Autodesk Inventor part; units mm, degrees
ref_plane "YZ Plane" through (0, 0, 0) normal (1, 0, 0) x (0, 1, 0)
ref_plane "XZ Plane" through (0, 0, 0) normal (0, 1, 0) x (-1, 0, 0)
ref_plane "XY Plane" through (0, 0, 0) normal (0, 0, 1) x (1, 0, 0)
sketch "Sketch1" plane through (0, 0, 0) normal (1, 0, 0) x (0, 1, 0)
  line L0 (0, 0) -> (-4.0897, 0)
  line L1 (0, -1.6442) -> (0, -13.25)
  line L2 (0, -13.25) -> (3.5, -13.25)
  line L3 (3.5, -13.25) -> (3.5, -10.75)
  line L4 (3.5, -10.75) -> (0.5, -10.75)
  line L5 (4, 0) -> (4, -10)
  line L6 (4, -10) -> (0.5, -10)
  line L7 (0.5, -10) -> (0.5, -10.75)
  line L8 (3.5, -1.5) -> (3.5, -9.5)
  line L9 (3.5, -9.5) -> (0, -9.5)
  line L10 (3, -11.25) -> (0, -11.25)
  line L11 (3, -11.25) -> (3, -12.25)
  line L12 (3, -12.25) -> (0, -12.25)
  line L13 (3.5, -1.5) -> (4, -1.5)
  point P0 (1.5, -12.25)
  point P1 (3.75, -1.5)
  dimension "d1" = 26.5
  dimension "d2" = 2.5
  dimension "d3" = 3.5
  dimension "d4" = 0
  dimension "d5" = 4
  dimension "d6" = 20
  dimension "d7" = 0.5
  dimension "d8" = 0.5
  dimension "d9" = 0.5
  dimension "d10" = 0.5
  dimension "d11" = 0.5
  dimension "d12" = 1
  dimension "d13" = 3
revolve "Revolution1" add sketch "Sketch1" angle 360 about axis through (0, 0, 0) along (0, -1, 0) contours L9 L8 L13 L5 L6 L7 L4 L3 L2 L1 L12 L11 L10
sketch "Sketch2" plane through (0, 4, 0) normal (0, 1, 0) x (1, 0, 0)
  line L0 (-7.75, 0) -> (7.75, 0)
  point P0 (0, 0)
  point P1 (0, 0)
  dimension "d15" = 15.5
hole "Hole1" at (-7.75, 4, 0) at (7.75, 4, 0) direction (0, -1, 0) diameter 1.5 end through all
fillet "Fillet1" radius 0.6 2 edges at (0, 0, 11.25) (0, 0, 9.5)
equation "\"d8\" = d7"
equation "\"d9\" = d7"
equation "\"d10\" = d7"
equation "\"d11\" = d7"
properties part number "Diaphram" material "Rubber, Silicone"
Can you work these out from the model? Positions are in its coordinate system, mm. A direction names the side the tool comes from. Coordinates: 2 decimals unless noted, no trailing zeros. Loops run counter-clockwise (first coordinate to the right, second up) from the corner with the lowest first, then second, coordinate; pieces in that order, holes last. Notation, with made-up numbers: M -40,47.25 L -33,47.25 A12 ccw -33,63.25 Z; hole C -23.5,41.5 d3. An arc over 180 degrees is marked long. Put each result on its own line as item: value. Start each with the question number.
(1) Will these pins go through, and if not, where does the flat tip stop? pin 1 Ø1.5 at (x, y) = (5, 0.5) entering from +Z; pin 2 Ø2.5 at (x, z) = (-7.75, 0) entering from -Y; pin 3 Ø2.5 at (x, z) = (0, 0) entering from +Y; pin 4 Ø1.5 at (x, y) = (1, 2) entering from -Z.
(2) We'd pull the mould along Z, two halves only. Please class faces 4 (the face through (-9.76, 2.23, 2.17)), 5 (the face through (0, 4, -2)), 6 (the face through (-11.172, 1.774, -7.123)): +Z half, -Z half, draft (parallel to the pull), parting line (faces both ways), or undercut.
(3) Which directions (+Z, -Z, +X, -X, +Y, -Y) give clear straight access to the entire face, cutting with the end or side of a thin tool? Please do faces 1 (the face through (-9, 0, -5)), 2 (the face through (-8.43, 2.03, -4.38)), 3 (the face through (-10, 0.5, -3)).
(4) Imagine slicing it at B-B on y = 2.55. List the corners of the cut face in (x, z) for me.
(5) I need wall thicknesses on probe 1 along X at (y, z) = (2.7, 0); probe 2 along X at (y, z) = (3.6, 0); probe 3 along Z at (x, y) = (4, 1). Which ranges of each line are inside material? Lowest first, please.
(6) Imagine slicing it at C-C on z = 0. Give the number of separate pieces and of enclosed holes in the cut face, and give its area (3 significant figures).
Worked answers:
1. pin 1: stops at z = 12.55
1. pin 2: stops at y = 3.5
1. pin 3: passes through
1. pin 4: stops at z = -13.25
2. face 4: undercut
2. face 5: draft
2. face 6: parting line
3. face 1: +Z, -Z, +X, -X, -Y
3. face 2: -Y
3. face 3: +Y
4. outline: C 0,0 d26.5; C 0,0 d22.5; C 0,0 d20; hole C 0,0 d24.5; hole C 0,0 d21.5; hole C 0,0 d19
5. probe 1: x = -13.25 to -12.25, -11.25 to -10.75, -10 to -9.5, 9.5 to 10, 10.75 to 11.25, 12.25 to 13.25
5. probe 2: x = -10 to -8.5, -7 to -1.5, 1.5 to 7, 8.5 to 10
5. probe 3: z = -12.63 to -11.58, -10.51 to -9.98, -9.17 to -8.62, 8.62 to 9.17, 9.98 to 10.51, 11.58 to 12.63
6. separate pieces: 4
6. enclosed holes: 0
6. area: 22.4 mm2
